```python
from build123d import *

# Parameters (mm, degrees)
CUT_EXTRUDE_START        = -1
CUT_EXTRUDE_1_DEPTH      = 1
PATTERN_CIRCULAR_1_COUNT = 3
FILLET_1_R               = 0.2


with BuildPart() as part:
    # Sketch 1 → Revolve 1 (revolve)
    with BuildSketch(Plane.XY, mode=Mode.PRIVATE) as revolve_1_sk:
        Polygon((-14.569649529, 2.696064574), (-14.569649529, 2.471705001), (-14.569649529, 0), (-16.769649529, 1.936980405), (-16.769649529, 2.471705001), (-15.719072987, 2.696064574), align=None)
    revolve(revolve_1_sk.sketch.rotate(Axis((-14.569649529, -1.803935426, 0), (-1, 0, 0)), 90), axis=Axis((-14.569649529, -1.803935426, 0), (-1, 0, 0)))

    # Sketch 6 → Cut-Extrude 1 (cut)
    with BuildSketch(Plane.ZY.offset(16.769649529).offset(CUT_EXTRUDE_START)):
        with BuildLine():
            Line((1.629390424, 1.293658293), (2.094930545, 2.17868507))
            ThreePointArc((2.094930545, 2.17868507), (2.434066949, 1.980944769), (2.754678634, 1.754399244))
            Line((2.754678634, 1.754399244), (2.142527827, 0.963658206))
            ThreePointArc((2.142527827, 0.963658206), (1.893163183, 1.139860281), (1.629390424, 1.293658293))
        make_face()
    cut_extrude_1 = extrude(amount=CUT_EXTRUDE_1_DEPTH, mode=Mode.SUBTRACT)

    # Pattern Circular 1: Cut-Extrude 1 ×3 about axis
    pattern_circular_1_axis = Axis((0, -1.803935426, 0), (1, 0, 0))
    for i in range(1, PATTERN_CIRCULAR_1_COUNT):
        add(cut_extrude_1.rotate(pattern_circular_1_axis, i * 360 / PATTERN_CIRCULAR_1_COUNT), mode=Mode.SUBTRACT)

    # Fillet 1
    fillet_1_edges = [part.edges().sort_by_distance(p)[0] for p in [
        (-16.769649529, -1.983103443, 3.736622817),
        (-16.769649529, -2.008713628, 4.270733771),
        (-16.769649529, 1.365574581, 2.453670694),
        (-16.769649529, 1.743498047, 1.866014286),
        (-16.769649529, -4.950361701, -2.023475463),
        (-16.769649529, -5.400110263, -2.312710011),
        (-16.769649529, -5.513631583, 1.518040837),
        (-16.769649529, -5.193667937, 2.139160363),
        (-16.769649529, 1.521658867, -1.713147354),
        (-16.769649529, 1.997017614, -1.95802376),
        (-15.719072987, -1.803935426, 4.5),
        (-16.769649529, -1.263749276, -3.971711531),
        (-16.769649529, -1.961636387, -4.005174649),
        (-14.569649529, -1.803935426, 4.5),
    ]]
    fillet(fillet_1_edges, radius=FILLET_1_R)


solid = part.part
```
Design review of the part built by this model. Coordinates are the model's own, in mm. A direction names the side the tool comes from. Give positions to 0.01 mm unless a question says otherwise; leave off trailing zeros. Write each loop counter-clockwise with the first axis right and the second up, starting at its lowest first coordinate (ties: lowest second). Pieces come first, ordered by that corner, then holes. Notation, with made-up numbers: (49.5, 72) - (102.5, 72) arc R14 cw to (102.5, 94) - close; hole circle Ø10 at (41, -38.5). An arc over 180 degrees is marked (long way). Return JSON: item names as keys, results as strings. Group by question number.
(1) Insertion check: pin 1 (0.5 mm diameter, centred on y = -5.5, z = 2, fed in from -X); pin 2 (1.2 mm diameter, centred on y = 1.5, z = 2, fed in from -X); pin 3 (2 mm diameter, centred on y = -1, z = -2.5, fed in from -X). Each pin has a flat end and moves straight along its axis. Give the tip position at first contact, or say it passes through.
(2) Mouldability with a two-part tool opening along Z and no side actions: class faces 4 (the flat face through (-16.16, -1.96, -3.98)), 5 (the flat face through (-16.16, -5.18, 2.13)), 6 (the cylindrical face through (-15.227, -0.08, -4.157)) as +Z half, -Z half, draft (parallel to the pull), parting line (faces both ways), or undercut.
(3) Machinability: for faces 1 (the flat face through (-15.77, 1.6, 2.2)), 2 (the flat face through (-16.164, -1.265, -3.965)), 3 (the flat face through (-14.57, -2, 2)), which of the approach directions +Z, -Z, +X, -X, +Y, -Y give a long, thin tool a straight path to every point of the face, cutting with its end or side? Answer none if there is none.
(4) We need section B-B, the plane x = -14.9. Give the boundary of the cut face in (y, z), then the cut area to 3 significant figures.
(5) We need section A-A, the plane x = -16.1. Give the boundary of the cut face in (y, z).
(6) To check wall thickness, follow probe 1 along X at (y, z) = (-1.75, -3.75); probe 2 along Y at (x, z) = (-15.3, 0); probe 3 along Z at (x, y) = (-14.9, -3.25). State the ranges of each line that lie inside material, in increasing order.
Reported:
{
 "1": {"pin 1": "stops at x = -15.77", "pin 2": "stops at x = -16.77", "pin 3": "stops at x = -16.64"},
 "2": {"face 4": "-Z half", "face 5": "undercut", "face 6": "parting line"},
 "3": {"face 1": "-X", "face 2": "-Z, -X", "face 3": "+Z, -Z, +X, +Y, -Y"},
 "4": {"outline": "circle Ø9 at (-1.8, 0); hole circle Ø4.19 at (-1.8, 0)", "area": "49.8 mm2"},
 "5": {"outline": "(-5.89, 1.67) arc R4.42 ccw to (-1.98, -4.42) - (-1.94, -3.5) arc R3.5 ccw to (-1.33, -3.47) - (-1.21, -4.38) arc R4.42 ccw to (2.11, 2.06) - (1.29, 1.63) arc R3.5 ccw to (0.96, 2.14) - (1.69, 2.7) arc R4.42 ccw to (-5.54, 2.36) - (-4.76, 1.87) arc R3.5 ccw to (-5.04, 1.33) - close; hole circle Ø6.3 at (-1.8, 0)"},
 "6": {"probe 1": "x = -15.77 to -14.57", "probe 2": "y = -6.3 to -4.25, 0.64 to 2.7", "probe 3": "z = -4.26 to -1.52, 1.52 to 4.26"}
}
